```python
from build123d import *

# Parameters (mm, degrees)
F0_W     = 177
F0_H     = 9
F1_DEPTH = 150
F2_W     = 400
F2_H     = 181
F2_R     = 3
F3_DEPTH = 9
F4_DEPTH = 150


with BuildPart() as f1:
    # F0 (on Front) → F1 (new body)
    with BuildSketch(Plane.XZ):
        Rectangle(F0_W, F0_H)
        with Locations((0, -86)):
            Rectangle(F0_W, F0_H)
        with Locations((0, 86)):
            Rectangle(F0_W, F0_H)
    extrude(amount=F1_DEPTH)

    # F2 (on face) → F3 (join)
    with BuildSketch(Plane(origin=(0, 0, 0), x_dir=(-1, 0, 0), z_dir=(0, 1, 0))):
        Rectangle(F2_W, F2_H)
        with Locations((-187, -50)):
            Circle(F2_R, mode=Mode.SUBTRACT)
        with Locations((187, -50)):
            Circle(F2_R, mode=Mode.SUBTRACT)
        with Locations((-187, 0)):
            Circle(F2_R, mode=Mode.SUBTRACT)
        with Locations((-187, 50)):
            Circle(F2_R, mode=Mode.SUBTRACT)
        with Locations((187, 0)):
            Circle(F2_R, mode=Mode.SUBTRACT)
        with Locations((187, 50)):
            Circle(F2_R, mode=Mode.SUBTRACT)
    extrude(amount=-F3_DEPTH)

    # F0 (on Front) → F4 (join)
    with BuildSketch(Plane.XZ):
        Polygon((-88.5, -81.5), (-88.5, -4.5), (-88.5, 4.5), (-88.5, 81.5), (-88.5, 90.5), (-97.5, 90.5), (-97.5, -90.5), (-88.5, -90.5), align=None)
        Polygon((88.5, 4.5), (88.5, -4.5), (88.5, -81.5), (88.5, -90.5), (97.5, -90.5), (97.5, 90.5), (88.5, 90.5), (88.5, 81.5), align=None)
    extrude(amount=F4_DEPTH)


solid = f1.part
```
Part model, mm, in its own coordinate system. A direction names the side the tool comes from. Round coordinates to 2 decimals unless told otherwise and drop trailing zeros. Write each loop counter-clockwise with the first axis right and the second up, starting at its lowest first coordinate (ties: lowest second). Pieces come first, ordered by that corner, then holes. Notation, with made-up numbers: M 63.5,-31 L 93.5,-31 A34 cw 93.5,1 Z; hole C 74.25,54.25 d9. An arc over 180 degrees is marked long. Answer as CSV lines item,"result". Start each with the question number.
1) Mould opens along X. For faces 4 (the face through (-1, -79, 4.5)), 5 (the face through (200, -4, -1)), 6 (the face through (-200, -4, -1)), 7 (the face through (-148, -9, 1)) say: +X half, -X half, draft (parallel to the pull), parting line (faces both ways), or undercut.
2) Drill centre lines: L1, parallel to Z at x = -187, y = -2; L2, parallel to Z at x = 33.5, y = -119.5; L3, parallel to X at y = -67, z = -37.5. Where is each one in solid material? Low to high.
3) Band-saw the part on D-D (x = -113.5). List the corners of the cut face in (y, z).
4) Band-saw the part on C-C (z = 12). List the corners of the cut face in (x, y), then the cut area to 3 significant figures.
5) Drop flat-ended pins along their axis: pin 1 (1 mm diameter, centred on y = -89.5, z = 64, fed in from -X); pin 2 (8 mm diameter, centred on y = -64.5, z = 58.5, fed in from +X); pin 3 (9.5 mm diameter, centred on x = -187, z = -50, fed in from +Y); pin 4 (7 mm diameter, centred on x = 187, z = 0, fed in from -Y). Give the stop position or say it passes through.
6) Band-saw the part on A-A (y = -111). List the corners of the cut face in (x, z), then the cut area to 3 significant figures.
7) Which spindle directions (+Z, -Z, +X, -X, +Y, -Y) get a long thin tool onto all of the face, cutting with end or side? Do faces 1 (the face through (-97.5, -79, 1)), 2 (the face through (149, -9, 1)), 3 (the face through (1, -9, -42)). Say none if no direction does.
8) Band-saw the part on B-B (x = 21.5). List the corners of the cut face in (y, z), then the cut area to 3 significant figures.
Worked out:
1,face 4,"undercut"
1,face 5,"+X half"
1,face 6,"-X half"
1,face 7,"draft"
2,L1,"-90.5 to -53, -47 to -3, 3 to 47, 53 to 90.5"
2,L2,"-90.5 to -81.5, -4.5 to 4.5, 81.5 to 90.5"
2,L3,"-97.5 to -88.5, 88.5 to 97.5"
3,outline,"M -9,-90.5 L 0,-90.5 L 0,90.5 L -9,90.5 Z"
4,outline,"M -200,-9 L -97.5,-9 L -97.5,-150 L -88.5,-150 L -88.5,-9 L 88.5,-9 L 88.5,-150 L 97.5,-150 L 97.5,-9 L 200,-9 L 200,0 L -200,0 Z"
4,area,"6,140 mm²"
5,pin 1,"x = -97.5"
5,pin 2,"x = 97.5"
5,pin 3,"y = 0"
5,pin 4,"y = -9"
6,outline,"M -97.5,-90.5 L 97.5,-90.5 L 97.5,90.5 L -97.5,90.5 Z; hole M -88.5,-81.5 L 88.5,-81.5 L 88.5,-4.5 L -88.5,-4.5 Z; hole M -88.5,4.5 L 88.5,4.5 L 88.5,81.5 L -88.5,81.5 Z"
6,area,"8,040 mm²"
7,face 1,"+Z, -Z, -X, -Y"
7,face 2,"+Z, -Z, +X, -Y"
7,face 3,"-Y"
8,outline,"M -150,-90.5 L 0,-90.5 L 0,90.5 L -150,90.5 L -150,81.5 L -9,81.5 L -9,4.5 L -150,4.5 L -150,-4.5 L -9,-4.5 L -9,-81.5 L -150,-81.5 Z"
8,area,"5,440 mm²"
